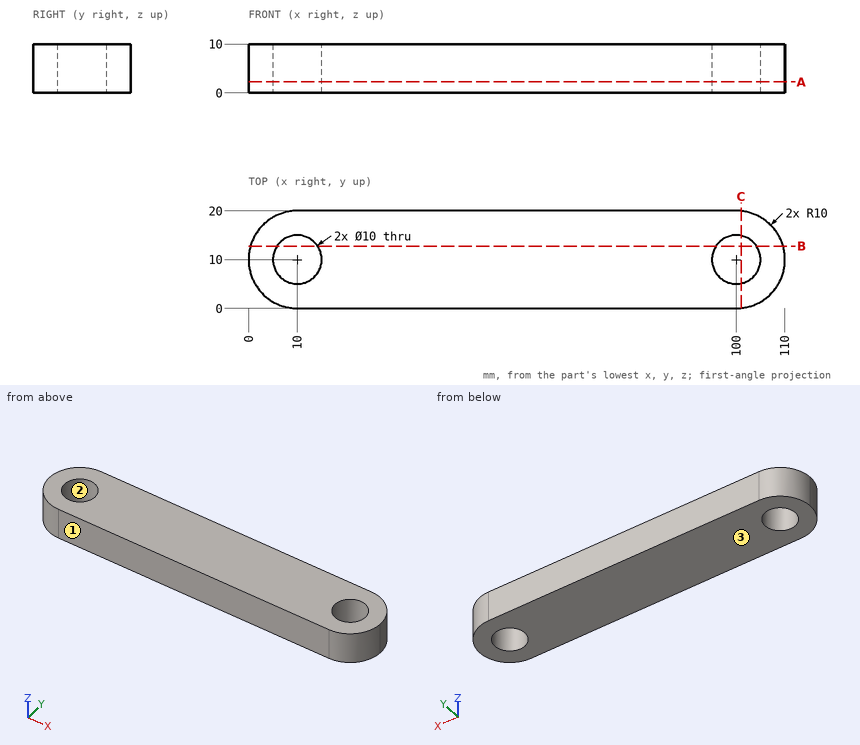
For this review, use the dimensioned drawing (mm, ordinates from the lowest corner) and the shaded views. Give positions to 0.01 mm unless a question says otherwise; leave off trailing zeros. Write each loop counter-clockwise with the first axis right and the second up, starting at its lowest first coordinate (ties: lowest second). Pieces come first, ordered by that corner, then holes. Notation, with made-up numbers: M 53.5,75 L 100.5,75 A30 cw 100.5,100 Z; hole C -8,52 d11. An arc over 180 degrees is marked long. Answer as a JSON object with one key per item and string values. Group by question number.
1) Clearance check with flat-ended pins moving along their axes: pin 1 Ø6 at (y, z) = (16, 5.5) entering from -X; pin 2 Ø1.5 at (y, z) = (8, 6.5) entering from -X. State where each tip first meets the part, or that it passes through.
2) We need section B-B (y = 12.75). Give the boundary of the cut face in (x, z), and give its area (3 significant figures).
3) We need section C-C (x = 101). Give the boundary of the cut face in (y, z).
4) We need section A-A (z = 2.25). Give the boundary of the cut face in (x, y), and give its area (3 significant figures).
5) For line 1 along X through (y, z) = (9.5, 3.25); line 2 along X through (y, z) = (6.25, 7); line 3 along Y through (x, z) = (104.5, 7.25), list the stretches that pass through material, from the lowest coordinate up.
6) Mouldability with a two-part tool opening along Y and no side actions: class the marked faces 1, 2 and 3 as released by +Y, released by -Y, zero draft, split by the parting line, or undercut.
Answer key:
{
 "1": {"pin 1": "stops at x = 0.46", "pin 2": "stops at x = 0.08"},
 "2": {"outline": "M 0.39,0 L 5.82,0 L 5.82,10 L 0.39,10 Z; M 14.18,0 L 95.82,0 L 95.82,10 L 14.18,10 Z; M 104.18,0 L 109.61,0 L 109.61,10 L 104.18,10 Z", "area": "925 mm²"},
 "3": {"outline": "M 0.05,0 L 5.1,0 L 5.1,10 L 0.05,10 Z; M 14.9,0 L 19.95,0 L 19.95,10 L 14.9,10 Z"},
 "4": {"outline": "M 0,10 A10 ccw 10,0 L 100,0 A10 ccw 110,10 A10 ccw 100,20 L 10,20 A10 ccw Z; hole C 10,10 d10; hole C 100,10 d10", "area": "1,960 mm²"},
 "5": {"line 1": "x = 0.01 to 5.03, 14.97 to 95.03, 104.97 to 109.99", "line 2": "x = 0.73 to 6.69, 13.31 to 96.69, 103.31 to 109.27", "line 3": "y = 1.07 to 7.82, 12.18 to 18.93"},
 "6": {"face 1": "released by -Y", "face 2": "undercut", "face 3": "zero draft"}
}
